from build123d import *

# Parameters (mm, degrees)
BOSS_EXTRUDE1_DEPTH = 8
CUT_EXTRUDE1_DEPTH  = 5.2
SKETCH3_R           = 2.3
BOSS_EXTRUDE2_DEPTH = 1
SKETCH4_R           = 1.25
CUT_EXTRUDE2_DEPTH  = 4.8
SKETCH5_R           = 1.5
SKETCH5_W           = 11
SKETCH5_H           = 10
CUT_EXTRUDE3_DEPTH  = 9
SKETCH7_R           = 0.6
BOSS_EXTRUDE3_DEPTH = 1.2


with BuildPart() as part:
    # Sketch1 → Boss-Extrude1 (new body)
    with BuildSketch(Plane(origin=(0, 0, 0), x_dir=(1, 0, 0), z_dir=(0, 1, 0))):
        with BuildLine():
            Line((5, 0), (40, 0))
            ThreePointArc((40, 0), (43.535533906, 1.464466094), (45, 5))
            Line((45, 5), (45, 20))
            ThreePointArc((45, 20), (43.535533906, 23.535533906), (40, 25))
            Line((40, 25), (5, 25))
            Line((5, 25), (0, 25))
            Line((0, 25), (0, 20))
            Line((0, 20), (0, 5))
            Line((0, 5), (0, 0))
            Line((0, 0), (5, 0))
        make_face()
    extrude(amount=BOSS_EXTRUDE1_DEPTH)

    # Sketch2 → Cut-Extrude1 (cut)
    with BuildSketch(Plane(origin=(0, 8, 0), x_dir=(1, 0, 0), z_dir=(0, 1, 0))):
        with BuildLine():
            Line((35.050927797, 15.15), (23.100878033, 14.49702088))
            ThreePointArc((23.100878033, 14.49702088), (21.21, 12.5), (23.100878033, 10.50297912))
            Line((23.100878033, 10.50297912), (35.050927797, 9.85))
            ThreePointArc((35.050927797, 9.85), (40.71, 12.5), (35.050927797, 15.15))
        make_face()
    extrude(amount=-CUT_EXTRUDE1_DEPTH, mode=Mode.SUBTRACT)

    # Sketch3 → Boss-Extrude2 (add)
    with BuildSketch(Plane(origin=(0, 2.8, 0), x_dir=(1, 0, 0), z_dir=(0, 1, 0))):
        with Locations((37.26, 12.5)):
            Circle(SKETCH3_R)
    extrude(amount=BOSS_EXTRUDE2_DEPTH)

    # Sketch4 → Cut-Extrude2 (cut, through all)
    with BuildSketch(Plane(origin=(0, 3.8, 0), x_dir=(1, 0, 0), z_dir=(0, 1, 0))):
        with Locations((37.26, 12.5)):
            Circle(SKETCH4_R)
    extrude(amount=-CUT_EXTRUDE2_DEPTH, mode=Mode.SUBTRACT)

    # Sketch5 → Cut-Extrude3 (cut, through all)
    with BuildSketch(Plane(origin=(0, 8, 0), x_dir=(1, 0, 0), z_dir=(0, 1, 0))):
        with Locations((5, 21.25)):
            Circle(SKETCH5_R)
        with Locations((5, 3.75)):
            Circle(SKETCH5_R)
        with Locations((5.5, 12.5)):
            Rectangle(SKETCH5_W, SKETCH5_H)
    extrude(amount=-CUT_EXTRUDE3_DEPTH, mode=Mode.SUBTRACT)

    # Sketch7 → Boss-Extrude3 (add)
    with BuildSketch(Plane(origin=(0, 2.8, 0), x_dir=(1, 0, 0), z_dir=(0, 1, 0))):
        with Locations((22.81, 12.5)):
            Circle(SKETCH7_R)
    extrude(amount=BOSS_EXTRUDE3_DEPTH)


solid = part.part
The listing builds one solid part. Answer for the finished solid, in the listing's coordinates (mm). A direction names the side the tool comes from. Round coordinates to 2 decimals unless told otherwise and drop trailing zeros. Order: outer loops, then holes, each group sorted by start corner. A loop starts at its lowest first (then second) coordinate and runs counter-clockwise, first axis right, second up. Notation, with made-up numbers: (8.5, 38) - (59.5, 38) arc R25 cw to (59.5, 73) - close; hole circle Ø5 at (11, 23). An arc over 180 degrees is marked (long way). Write item = value, one per line. Start each with the question number.
1) Section A-A, the plane z = -12.5 is taken. Write down the section's boundary in (x, y).
2) Section C-C, the plane x = 37.26 is taken. Write down the section's boundary in (y, z), plus the area to 3 significant figures.
3) Section B-B, the plane y = 3.25 is taken. Write down the section's boundary in (x, z).
4) Given pin 1 (2 mm diameter, centred on x = 37.26, z = -12.5, fed in from -Y); pin 2 (2 mm diameter, centred on x = 32.5, z = -12, fed in from +Y); pin 3 (2.5 mm diameter, centred on x = 37, z = -13, fed in from +Y); pin 4 (1 mm diameter, centred on y = 1, z = -22, fed in from +X), each flat-ended and moving along its own axis, determine where each tip first touches the part or whether it passes through.
5) For faces 1 (the flat face through (20, 4, 0)), 2 (the flat face through (22.8, 4, -12.5)), determine the directions among +Z, -Z, +X, -X, +Y, -Y from which every point of the face is accessible in a straight line to the end or side of a thin tool.
6) Section D-D, the plane y = 7.5 is taken. Write down the section's boundary in (x, z), plus the area to 3 significant figures.
7) Straight lines are drawn through the part: L1, parallel to Z at x = 5, y = 2; L2, parallel to Z at x = 37.26, y = 2.15; L3, parallel to Z at x = 35, y = 4.5. For each, find the intervals that lie inside material, in ascending order.
8) For a pull along Z with two mould halves and no side action, classify faces 3 (the flat face through (29.16, 5.44, -14.83)), 4 (the flat face through (22, 8, -15)), 5 (the cylindrical face through (43, 4, -1)) as released by +Z, released by -Z, zero draft, split by the parting line, or undercut.
Results list:
q1.outline = (11, 0) - (36.01, 0) - (36.01, 3.8) - (34.96, 3.8) - (34.96, 2.8) - (23.41, 2.8) - (23.41, 4) - (22.21, 4) - (22.21, 2.8) - (21.21, 2.8) - (21.21, 8) - (11, 8) - close; (38.51, 0) - (45, 0) - (45, 8) - (40.71, 8) - (40.71, 2.8) - (39.56, 2.8) - (39.56, 3.8) - (38.51, 3.8) - close
q2.outline = (0, -25) - (8, -25) - (8, -15.95) - (2.8, -15.95) - (2.8, -14.8) - (3.8, -14.8) - (3.8, -13.75) - (0, -13.75) - close; (0, -11.25) - (3.8, -11.25) - (3.8, -10.2) - (2.8, -10.2) - (2.8, -9.05) - (8, -9.05) - (8, 0) - (0, 0) - close
q2.area = 159 mm^2
q3.outline = (0, -25) - (40, -25) arc R5 ccw to (45, -20) - (45, -5) arc R5 ccw to (40, 0) - (0, 0) - (0, -7.5) - (11, -7.5) - (11, -17.5) - (0, -17.5) - close; circle Ø1.2 at (22.81, -12.5); circle Ø4.6 at (37.26, -12.5); hole circle Ø3 at (5, -21.25); hole circle Ø3 at (5, -3.75); hole (23.1, -14.5) - (35.05, -15.15) arc R3.45 ccw (long way) to (35.05, -9.85) - (23.1, -10.5) arc R2 ccw to start; hole circle Ø2.5 at (37.26, -12.5)
q4.pin_1 = through
q4.pin_2 = 2.8
q4.pin_3 = 3.8
q4.pin_4 = 44.77
q5.face_1 = +Z, +X, -X, +Y, -Y
q5.face_2 = +Y
q6.outline = (0, -25) - (40, -25) arc R5 ccw to (45, -20) - (45, -5) arc R5 ccw to (40, 0) - (0, 0) - (0, -7.5) - (11, -7.5) - (11, -17.5) - (0, -17.5) - close; hole circle Ø3 at (5, -21.25); hole circle Ø3 at (5, -3.75); hole (23.1, -14.5) - (35.05, -15.15) arc R3.45 ccw (long way) to (35.05, -9.85) - (23.1, -10.5) arc R2 ccw to start
q6.area = 896 mm^2
q7.L1 = -25 to -22.75, -19.75 to -17.5, -7.5 to -5.25, -2.25 to 0
q7.L2 = -25 to -13.75, -11.25 to 0
q7.L3 = -25 to -15.15, -9.85 to 0
q8.face_3 = undercut
q8.face_4 = zero draft
q8.face_5 = released by +Z
